Autodesk Inventor part; units mm, degrees
ref_plane "YZ Plane" through (0, 0, 0) normal (1, 0, 0) x (0, 1, 0)
ref_plane "XZ Plane" through (0, 0, 0) normal (0, 1, 0) x (-1, 0, 0)
ref_plane "XY Plane" through (0, 0, 0) normal (0, 0, 1) x (1, 0, 0)
sketch "Sketch1" plane through (0, 0, 0) normal (0, 0, 1) x (1, 0, 0)
  line L0 (0, 0) -> (0, 7.5879)
  line L1 (-24.0284, 0) -> (-24.0284, 11.557)
  line L2 (-24.0284, 11.557) -> (-4, 11.557)
  line L3 (-4, 11.557) -> (-4, 0)
  line L4 (-24.0284, 0) -> (-4, 0)
  dimension "d0" = 48.0568
  dimension "d2" = 8
  dimension "d3" = 11.557
revolve "Revolution1" add sketch "Sketch1" angle 360 about axis through (0, 0, 0) along (0, 1, 0)
fillet "Fillet1" radius 3.175 1 edges at (24.0284, 11.557, 0)
chamfer "Chamfer1" distance 3.175 angle 45 1 edges at (4, 0, 0)
properties part number "SMALL-MAGNET" material "Steel, Alloy"
Model file for the job. Use its own axes, mm. Round coordinates to 2 decimals unless told otherwise and drop trailing zeros. Loops run counter-clockwise (first coordinate to the right, second up) from the corner with the lowest first, then second, coordinate; pieces in that order, holes last. Notation, with made-up numbers: M 5.5,12 L 13.5,12 A21 ccw 13.5,42 Z; hole C -6.5,42 d11. An arc over 180 degrees is marked long. Put each result on its own line as item: value. Start each with the question number.
Item 1: Cut at D-D (y = 1). List the corners of the cut face in (x, z) (3 decimals).
Item 2: Drop flat-ended pins along their axis: P1, Ø1, axis at y = 3.5, z = -17.5, coming from the +X side; P2, Ø1.5, axis at y = 10, z = -7.5, coming from the +X side; P3, Ø10.5, axis at x = 0, z = 0, coming from the -Y side (3 decimals). Give the stop position or say it passes through.
Item 3: Drill centre lines: line 1 along Z through (x, y) = (-2.5, 8); line 2 along Z through (x, y) = (-3, 1.75); line 3 along X through (y, z) = (3, -1.5). Where is each one in solid material? Low to high.
Item 4: Mould opens along Z. For faces 1 (the face through (0.867, 7.307, 3.905)), 2 (the face through (-5, 0, 6)), 3 (the face through (5.209, 4.25, -23.457)), 4 (the face through (0.91, 2.976, 4.099)) say: released by +Z, released by -Z, zero draft, split by the parting line, or undercut.
Item 5: Cut at A-A (x = 0). List the corners of the cut face in (y, z) (3 decimals), then the cut area to 3 significant figures.
Item 6: Cut at B-B (z = 0). List the corners of the cut face in (x, y) (3 decimals), then the cut area to 3 significant figures.
Item 7: Cut at C-C (y = 4.25). List the corners of the cut face in (x, z).
Answer block:
1. outline: C 0,0 d48.057; hole C 0,0 d12.35
2. P1: x = 16.98
2. P2: x = 22.8
2. P3: y = 1.925
3. line 1: -23.9 to -3.12, 3.12 to 23.9
3. line 2: -23.84 to -4.52, 4.52 to 23.84
3. line 3: -23.98 to -3.9, 3.9 to 23.98
4. face 1: undercut
4. face 2: zero draft
4. face 3: split by the parting line
4. face 4: undercut
5. outline: M 0,-24.028 L 8.382,-24.028 A3.175 ccw 11.557,-20.853 L 11.557,-4 L 3.175,-4 L 0,-7.175 Z; M 0,7.175 L 3.175,4 L 11.557,4 L 11.557,20.853 A3.175 ccw 8.382,24.028 L 0,24.028 Z
5. area: 449 mm2
6. outline: M -24.028,0 L -7.175,0 L -4,3.175 L -4,11.557 L -20.853,11.557 A3.175 ccw -24.028,8.382 Z; M 4,3.175 L 7.175,0 L 24.028,0 L 24.028,8.382 A3.175 ccw 20.853,11.557 L 4,11.557 Z
6. area: 449 mm2
7. outline: C 0,0 d48.06; hole C 0,0 d8
